Geometry check sheet. Reference: the model listing, model coordinates, mm. A direction names the side the tool comes from. Give positions to 0.01 mm unless a question says otherwise; leave off trailing zeros. Write each loop counter-clockwise with the first axis right and the second up, starting at its lowest first coordinate (ties: lowest second). Pieces come first, ordered by that corner, then holes. Notation, with made-up numbers: (35, 21) - (51, 21) arc R11 ccw to (51, 37) - close; hole circle Ø8 at (51, -3). An arc over 180 degrees is marked (long way). One line per question, with ' | ' between items. Start each with the question number.
Q1. Section check B-B on x = 0. Record the boundary of the cut face in (y, z).
Q2. Release check for a two-part mould opening along Y. For faces 1 (the face through (0, -4, 0)), 2 (the face through (0, 3, 19)), 3 (the face through (0, 0, -3)), 4 (the face through (0, 0, 3)) record: +Y half, -Y half, draft (parallel to the pull), parting line (faces both ways), or undercut.
Q3. Gauge pin test, flat ends, axial feed: P1, Ø1.5, axis at x = 1, y = -2, coming from the -Z side; P2, Ø2, axis at x = 0, y = 0, coming from the +Z side; P3, Ø1.5, axis at x = 2, y = 2, coming from the +Z side. Record the tip position at first contact, or that the pin passes through.
Q4. Section check D-D on y = 0.25. Record the boundary of the cut face in (x, z), and give its area (3 significant figures).
Q5. Section check C-C on y = -3. Record the boundary of the cut face in (x, z), and give its area (3 significant figures).
Q6. Thickness scan on L1, parallel to Z at x = 0, y = -3.15; L2, parallel to Y at x = 0.5, z = -17; L3, parallel to Z at x = 1.75, y = 3. Record the ranges inside material, lowest first. Write a range as [from, to].
Q7. Section check A-A on z = 7. Record the boundary of the cut face in (x, y), and give its area (3 significant figures).
Q8. Set-up check for faces 5 (the face through (3.4, 0.03, 2.43)), 6 (the face through (-3.43, -0.03, -2.4)), 7 (the face through (3.43, 0.03, -2.4)), 8 (the face through (-3.4, -0.03, 2.43)): record each of +Z, -Z, +X, -X, +Y, -Y from which the full face is reachable in a straight line by a thin tool's end or side.
Autodesk Inventor part; units mm, degrees
ref_plane "YZ Plane" through (0, 0, 0) normal (1, 0, 0) x (0, 1, 0)
ref_plane "XZ Plane" through (0, 0, 0) normal (0, 1, 0) x (-1, 0, 0)
ref_plane "XY Plane" through (0, 0, 0) normal (0, 0, 1) x (1, 0, 0)
sketch "Szkic1" plane through (0, 0, 0) normal (0, 1, 0) x (-1, 0, 0)
  line L0 (0, 15) -> (0, -15) construction
  line L1 (-4, 15) -> (-4, -15)
  line L2 (4, -15) -> (4, 15)
  arc A0 (4, 15) -> (-4, 15) centre (0, 15) ccw
  arc A1 (-4, -15) -> (4, -15) centre (0, -15) ccw
  circle A2 centre (0, -15) radius 2
  circle A3 centre (0, 15) radius 2
  line L3 (0, 15) -> (0, 3)
  line L4 (0, 3) -> (4, 3)
  line L5 (0, 3) -> (-4, 3)
  point P0 (0, 0)
  dimension "d0" = 15
  dimension "d1" = 8
  dimension "d2" = 4
  dimension "d3" = 4
  dimension "d6" = 12
extrude "Wyciągnięcie proste1" add sketch "Szkic1" along normal mid plane 8 contours A0 L2 L4 L5 L1 | L5 L4 L2 A1 L1 | A2 | A3
extrude "Wyciągnięcie proste2" cut sketch "Szkic1" along normal mid plane 4 contours A0 L2 L4 L5 L1
extrude "Wyciągnięcie proste3" cut sketch "Szkic1" along normal mid plane 14.5 contours A3
mirror "Odbij1" about plane through (0, 0, 0) normal (0, 0, 1) of "Wyciągnięcie proste2", "Wyciągnięcie proste3"
fillet "Zaokrąglenie1" radius 2 4 edges at (-4, 0, 3) (-4, 0, -3) (4, 0, -3) (4, 0, 3)
properties part number "connector"
Working result:
1) outline: (-4, -19) - (-2, -19) - (-2, -17) - (-4, -17) - close; (-4, -13) - (-2, -13) - (-2, -3) - (2, -3) - (2, -13) - (4, -13) - (4, 13) - (2, 13) - (2, 3) - (-2, 3) - (-2, 13) - (-4, 13) - close; (-4, 17) - (-2, 17) - (-2, 19) - (-4, 19) - close; (2, -19) - (4, -19) - (4, -17) - (2, -17) - close; (2, 17) - (4, 17) - (4, 19) - (2, 19) - close
2) face 1: -Y half | face 2: draft | face 3: undercut | face 4: undercut
3) P1: stops at z = -18.99 | P2: stops at z = 3 | P3: stops at z = 18.8
4) outline: (-4, -1) arc R2 ccw to (-2, -3) - (2, -3) arc R2 ccw to (4, -1) - (4, 1) arc R2 ccw to (2, 3) - (-2, 3) arc R2 ccw to (-4, 1) - close | area: 44.6 mm2
5) outline: (-4, -15) arc R4 ccw to (4, -15) - (4, 15) arc R4 ccw to (-4, 15) - close; hole circle Ø4 at (0, -15); hole circle Ø4 at (0, 15) | area: 265 mm2
6) L1: z = [-19, -17], [-13, 13], [17, 19] | L2: y = [-4, -2], [2, 4] | L3: z = [-18.6, -15.97], [-14.03, 14.03], [15.97, 18.6]
7) outline: (-4, -4) - (4, -4) - (4, -2) - (-4, -2) - close; (-4, 2) - (4, 2) - (4, 4) - (-4, 4) - close | area: 32.0 mm2
8) face 5: +Z, +X | face 6: -Z, -X | face 7: -Z, +X | face 8: +Z, -X
